Study the drawing (mm; zero at the part's minimum x, y, z) and answer. A direction names the side the tool comes from. Give positions to 0.01 mm unless a question says otherwise; leave off trailing zeros. Order: outer loops, then holes, each group sorted by start corner. A loop starts at its lowest first (then second) coordinate and runs counter-clockwise, first axis right, second up.
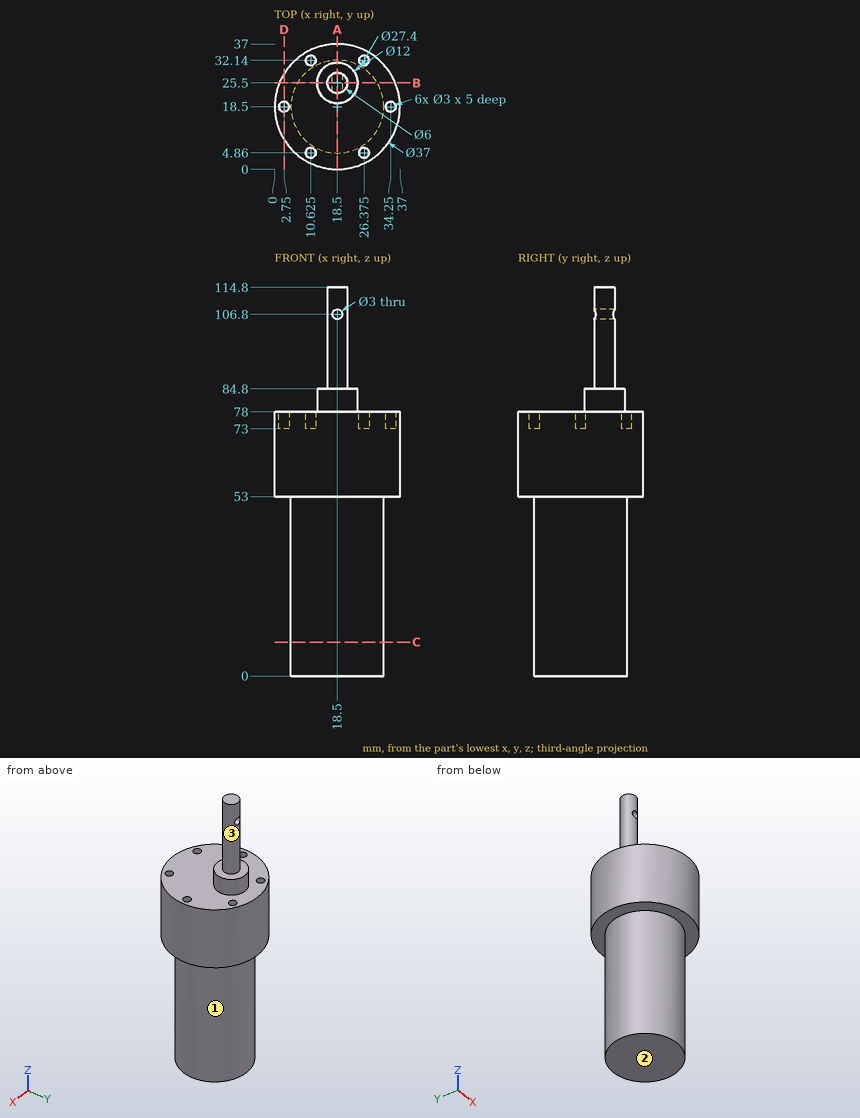
1) Find section B-B (y = 25.5). Write down the section's boundary in (x, z).
Geometry says:
outline: (1.38, 53) - (6.72, 53) - (6.72, 0) - (30.28, 0) - (30.28, 53) - (35.62, 53) - (35.62, 78) - (24.5, 78) - (24.5, 84.8) - (21.5, 84.8) - (21.5, 114.8) - (15.5, 114.8) - (15.5, 84.8) - (12.5, 84.8) - (12.5, 78) - (1.38, 78) - close; hole circle Ø3 at (18.5, 106.8)
2) Find section A-A (x = 18.5). Write down the section's boundary in (y, z), then the cut area to 3 significant figures.
Geometry says:
outline: (0, 53) - (4.8, 53) - (4.8, 0) - (32.2, 0) - (32.2, 53) - (37, 53) - (37, 78) - (31.5, 78) - (31.5, 84.8) - (28.5, 84.8) - (28.5, 105.3) - (22.5, 105.3) - (22.5, 84.8) - (19.5, 84.8) - (19.5, 78) - (0, 78) - close; (22.5, 108.3) - (28.5, 108.3) - (28.5, 114.8) - (22.5, 114.8) - close
area: 2,620 mm2
3) Find section D-D (x = 2.75). Write down the section's boundary in (y, z) (3 decimals).
Geometry says:
outline: (8.795, 53) - (28.205, 53) - (28.205, 78) - (20, 78) - (20, 73) - (17, 73) - (17, 78) - (8.795, 78) - close
4) Find section C-C (z = 10). Write down the section's boundary in (x, y).
Geometry says:
outline: circle Ø27.4 at (18.5, 18.5)
5) Given P1, Ø1.5, axis at y = 20.5, z = 28, coming from the -X side; P2, Ø18.5, axis at x = 18, y = 22, coming from the -Z side; P3, Ø2.5, axis at x = 18.5, z = 106.8, coming from the -Y side; P4, Ø3, axis at x = 22, y = 18.5, coming from the +Z side, each flat-ended and moving along its own axis, determine where each tip first touches the part or whether it passes through.
Geometry says:
P1: stops at x = 4.86
P2: stops at z = 0
P3: passes through
P4: stops at z = 78
6) Straight lines are drawn through the part: probe 1 along Z at (x, y) = (31.5, 17.5); probe 2 along Z at (x, y) = (22.5, 33.5); probe 3 along Y at (x, z) = (18.5, 91.5). For each, find the intervals that lie inside material, in ascending order.
Geometry says:
probe 1: z = 0 to 78
probe 2: z = 53 to 78
probe 3: y = 22.5 to 28.5
7) A tool of negligible diameter and unlimited length cuts with its end or side. For the marked faces 1, 2 and 3, from which of +Z, -Z, +X, -X, +Y, -Y can it reach the whole face along a straight path? Write none if from no direction.
Geometry says:
face 1: -Z
face 2: -Z, +X, -X, +Y, -Y
face 3: +Z
